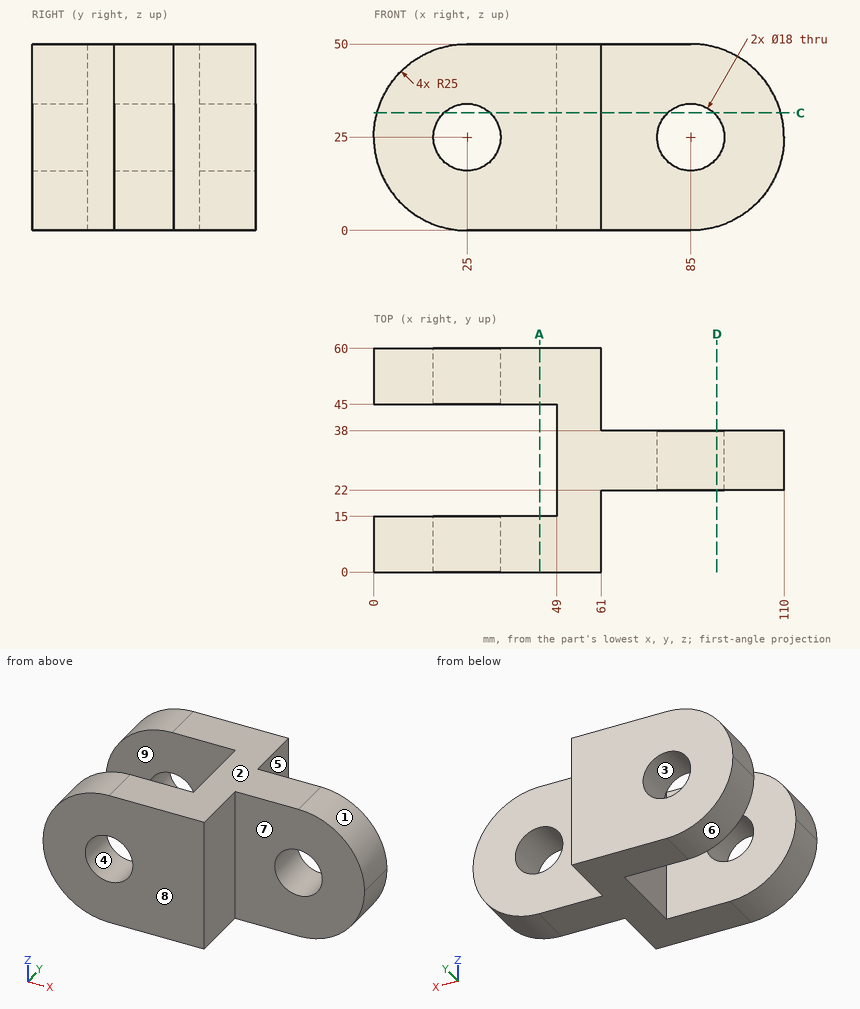
Input: dimensioned drawing with shaded views. Units: mm. Origin: part minimum x, y, z. A direction names the side the tool comes from. Give positions to 0.01 mm unless a question says otherwise; leave off trailing zeros. Loops run counter-clockwise (first coordinate to the right, second up) from the corner with the lowest first, then second, coordinate; pieces in that order, holes last. Notation, with made-up numbers: M 31,42 L 66,42 A19 ccw 66,66 Z; hole C 88,5 d7. An arc over 180 degrees is marked long. Put each result on its own line as item: value.
1) Mould query, pull axis X, two halves, no side actions, for the marked faces 1, 2, 3 and 4. Classes: released by +X, released by -X, zero draft, split by the parting line, or undercut.
Computed values:
face 1: released by +X
face 2: zero draft
face 3: undercut
face 4: undercut
2) First-contact query: P1, Ø6, axis at x = 24, z = 18, coming from the -Y side; P2, Ø5, axis at y = 21, z = 10.5, coming from the -X side; P3, Ø1, axis at x = 79.5, z = 18, coming from the -Y side; P4, Ø14.5, axis at x = 93.5, z = 20.5, coming from the +Y side. Flat tips, straight axial feed; report the tip coordinate or a pass-through.
Computed values:
P1: stops at y = 0
P2: stops at x = 49
P3: stops at y = 22
P4: stops at y = 38
3) Reachability of the marked faces 5, 6, 7, 8 and 9 from +Z, -Z, +X, -X, +Y, -Y: full face, straight path, thin tool, end or side. Return the list, or none.
Computed values:
face 5: +Z, -Z, +X, +Y
face 6: -Z, -X, +Y, -Y
face 7: +Z, -Z, +X, -Y
face 8: +Z, -Z, +X, -X, -Y
face 9: +Z, -Z, -X
4) Cut plane A-A, the plane x = 44.5. Return the cut outline in (y, z).
Computed values:
outline: M 0,0 L 15,0 L 15,50 L 0,50 Z; M 45,0 L 60,0 L 60,50 L 45,50 Z
5) Material intervals for L1, parallel to Y at x = 25, z = 4; L2, parallel to X at y = 49.5, z = 25; L3, parallel to Y at x = 72, z = 48, sorted ascending. Write a range as from..to.
Computed values:
L1: y = 0..15, 45..60
L2: x = 0..16, 34..61
L3: y = 22..38
6) Cut plane C-C, the plane z = 31.5. Return the cut outline in (x, y) (1 decimal).
Computed values:
outline: M 0.9,0 L 18.8,0 L 18.8,15 L 0.9,15 Z; M 0.9,45 L 18.8,45 L 18.8,60 L 0.9,60 Z; M 31.2,0 L 61,0 L 61,22 L 78.8,22 L 78.8,38 L 61,38 L 61,60 L 31.2,60 L 31.2,45 L 49,45 L 49,15 L 31.2,15 Z; M 91.2,22 L 109.1,22 L 109.1,38 L 91.2,38 Z
7) Cut plane D-D, the plane x = 92. Return the cut outline in (y, z).
Computed values:
outline: M 22,1 L 38,1 L 38,19.34 L 22,19.34 Z; M 22,30.66 L 38,30.66 L 38,49 L 22,49 Z
